Source: CAD feature listing. Evaluate the final solid. Frame: model axes, mm. A direction names the side the tool comes from. Give positions to 0.01 mm unless a question says otherwise; leave off trailing zeros. Order: outer loops, then holes, each group sorted by start corner. A loop starts at its lowest first (then second) coordinate and runs counter-clockwise, first axis right, second up. Notation, with made-up numbers: (54.5, -33) - (103.5, -33) arc R22 cw to (103.5, -24) - close; hole circle Ø8 at (61, -11.5). An arc over 180 degrees is marked (long way). Write each question's results on one line, items separated by ' | '. Start each with the question number.
Item 1: Contact query for flat-ended pins moving along their axis: pin 1 Ø1.9 at (y, z) = (9, 17) entering from -X; pin 2 Ø9.5 at (x, y) = (-1, 19) entering from +Z; pin 3 Ø3 at (x, z) = (-15, 51) entering from -Y. Output: stop coordinate, or through.
Item 2: Section B-B on z = -1.5. Output: boundary loops of the cut face in (x, y), and give its area (3 significant figures).
Item 3: Set-up query: faces 1 (the cylindrical face through (36.23, -0.178, 38.416)), 2 (the flat face through (50, 0, 43.381)), 3 (the flat face through (31.522, 0, 5)), 4 (the flat face through (-2, 6.35, 36)), 5 (the flat face through (12.472, -10, 18)). Return all of +Z, -Z, +X, -X, +Y, -Y with unobstructed straight access to the full face (end or side cutting, diameter ignored); none if empty.
Item 4: Section A-A on x = 52.5. Output: boundary loops of the cut face in (y, z).
Item 5: Line query: line 1 along Z through (x, y) = (-7, -17.5); line 2 along Y through (x, z) = (-20, 31); line 3 along Y through (x, z) = (21, 23). Output: solid intervals per line, ascending.
```python
from build123d import *

# Parameters (mm, degrees)
F1_DEPTH = 25.4
F0_W     = 25.4
F0_H     = 19.05
F2_DEPTH = 12.7
F4_DEPTH = 6.35


with BuildPart() as f1:
    # F0 (on Front) → F1 (new body, symmetric)
    with BuildSketch(Plane.XZ):
        Polygon((31.5217984643, -9.0189850047), (31.5217984643, 9.0189850047), (12.4717984643, 9.0189850047), (-31.5217984643, 9.0189850047), (-31.5217984643, -9.0189850047), align=None)
    extrude(amount=F1_DEPTH, both=True)

    # F0 (on Front) → F2 (join, symmetric)
    with BuildSketch(Plane.XZ):
        with BuildLine():
            Line((12.4717984643, 9.0189850047), (31.5217984643, 9.0189850047))
            Line((31.5217984643, 9.0189850047), (31.5217984643, 26.8712149953))
            ThreePointArc((31.5217984643, 26.8712149953), (36.3574655069, 38.5455479527), (48.0317984643, 43.3812149953))
            Line((48.0317984643, 43.3812149953), (50.5717984643, 43.3812149953))
            Line((50.5717984643, 43.3812149953), (50.5717984643, 62.4312149953))
            Line((50.5717984643, 62.4312149953), (48.0317984643, 62.4312149953))
            add(Edge.make_bspline(
                [(46.7575546459, 62.4083772721), (47.1808590375, 62.4161488041), (47.6056092378, 62.4237507503), (48.0317984643, 62.4312149953)],
                knots=[94.9706554632, 94.9706554632, 94.9706554632, 94.9706554632, 95.8208802759, 95.8208802759, 95.8208802759, 95.8208802759], degree=3))
            ThreePointArc((46.7575546459, 62.4083772721), (22.4405332535, 51.5613090597), (12.4717984643, 26.8712149953))
            Line((12.4717984643, 26.8712149953), (12.4717984643, 9.0189850047))
        make_face()
        with Locations((63.2717984643, 52.9062149953)):
            Rectangle(F0_W, F0_H)
    extrude(amount=F2_DEPTH, both=True)

    # F0 (on Front) → F3 (revolve)
    with BuildSketch(Plane.XZ):
        Polygon((75.9717984643, 62.4312149953), (75.9717984643, 43.3812149953), (75.9717984643, 38.6187149953), (101.3717984643, 38.6187149953), (101.3717984643, 67.1937149953), (75.9717984643, 67.1937149953), align=None)
    revolve(axis=Axis((75.9717984643, 0, 52.9062149953), (0, 0, -1)))

    # F0 (on Front) → F4 (join, symmetric)
    with BuildSketch(Plane.XZ):
        with BuildLine():
            Line((-31.5217984643, 9.0189850047), (12.4717984643, 9.0189850047))
            Line((12.4717984643, 9.0189850047), (12.4717984643, 26.8712149953))
            ThreePointArc((12.4717984643, 26.8712149953), (22.4405332535, 51.5613090597), (46.7575546459, 62.4083772721))
            add(Edge.make_bspline(
                [(-31.5217984643, 9.0189850047), (-29.7697852659, 58.5562793016), (-0.5258166747, 61.5402921774), (46.7575546459, 62.4083772721)],
                knots=[0, 0, 0, 0, 94.9706554632, 94.9706554632, 94.9706554632, 94.9706554632], degree=3))
        make_face()
    extrude(amount=F4_DEPTH, both=True)


solid = f1.part
```
Evaluation:
1) pin 1: stops at x = 12.47 | pin 2: stops at z = 9.02 | pin 3: stops at y = -6.35
2) outline: (-31.52, -25.4) - (31.52, -25.4) - (31.52, 25.4) - (-31.52, 25.4) - close | area: 3,200 mm^2
3) face 1: -Z, +Y, -Y | face 2: -Z | face 3: -Z, +X, +Y, -Y | face 4: +Z, -X, +Y | face 5: +Z, -X, -Y
4) outline: (-12.7, 43.38) - (-9.71, 43.38) - (-9.71, 38.62) - (9.71, 38.62) - (9.71, 43.38) - (12.7, 43.38) - (12.7, 62.43) - (9.71, 62.43) - (9.71, 67.19) - (-9.71, 67.19) - (-9.71, 62.43) - (-12.7, 62.43) - close
5) line 1: z = -9.02 to 9.02 | line 2: y = -6.35 to 6.35 | line 3: y = -12.7 to 12.7
